Read the model definition and answer for the solid it produces. Units are mm, in the model's axes. Face numbers are marked on the shaded views. A direction names the side the tool comes from. Round coordinates to 2 decimals unless told otherwise and drop trailing zeros. Write each loop counter-clockwise with the first axis right and the second up, starting at its lowest first coordinate (ties: lowest second). Pieces come first, ordered by that corner, then holes. Notation, with made-up numbers: (3.5, 23.5) -> (12.5, 23.5) arc R33 ccw to (12.5, 60.5) -> close; hole circle Ø10 at (24.25, 84). An arc over 180 degrees is marked (long way). Return JSON: item names as keys, results as strings. Group by question number.
(1) For the marked faces 1 and 2, determine the directions among +Z, -Z, +X, -X, +Y, -Y from which every point of the face is accessible in a straight line to the end or side of a thin tool.
(2) Straight lines are drawn through the part: line 1 (Y direction, x = 0, z = 0.55); line 2 (X direction, y = 26, z = 0); line 3 (Y direction, x = -34.5, z = -0.65). For each, find the intervals that lie inside material, in ascending order.
(3) A cutting plane is placed at A-A on z = -0.75. Give the vertices of the cut face in (x, y), then the cut area to 3 significant figures.
(4) A cutting plane is placed at C-C on y = 22. State how many separate pieces and enclosed holes the cut face has, then the cut area to 3 significant figures.
(5) The mould has two halves that part along X. Classify the marked faces 3 and 4: released by +X, released by -X, zero draft, split by the parting line, or undercut.
(6) Given pin 1 (1 mm diameter, centred on y = -26, z = -2, fed in from -X); pin 2 (1 mm diameter, centred on y = -8, z = 0, fed in from -X); pin 3 (1.5 mm diameter, centred on y = -19.5, z = -2, fed in from +X), each flat-ended and moving along its own axis, determine where each tip first touches the part or whether it passes through.
(7) A cutting plane is placed at B-B on x = 0. Give the vertices of the cut face in (y, z), then the cut area to 3 significant figures.
```python
from build123d import *

# Parameters (mm, degrees)
CENTER_REACH             = 60.766
SKETCH3_R                = 7.5
CENTER_DIRECTION_2_REACH = 60.766
SPOKES_DEPTH             = 6
SKETCH5_R                = 2.75
HOLE_DEPTH               = 6


with BuildPart() as part:
    # Sketch2 → rim (revolve)
    with BuildSketch(Plane(origin=(0, 0, 0), x_dir=(1, 0, 0), z_dir=(0, 1, 0)), mode=Mode.PRIVATE) as rim_sk:
        with BuildLine():
            Line((41.5, -1.78), (41.5, -3))
            Line((41.5, -3), (38, -3))
            Line((38, -3), (38, 3))
            Line((38, 3), (41.5, 3))
            Line((41.5, 3), (41.5, 1.78))
            ThreePointArc((41.5, 1.78), (39.72, 0), (41.5, -1.78))
        make_face()
    revolve(rim_sk.sketch.rotate(Axis((0, 0, -19.925351406), (0, 0, 1)), 180), axis=Axis((0, 0, -19.925351406), (0, 0, 1)))


with BuildPart() as body_2:

    # center: up to this face of the body (flat: up to its plane)
    center_end = Plane(part.part.faces().sort_by_distance((40.326202743, 0, 3))[0])
    # Sketch3 → center (new, up to the picked face)
    with BuildSketch(Plane.XY, mode=Mode.PRIVATE) as center_sk1:
        with Locations(Location((0, 0, 0), (0, 0, 180))):
            Circle(SKETCH3_R)
    center_tool1 = split(extrude(center_sk1.sketch, amount=CENTER_REACH, mode=Mode.PRIVATE), bisect_by=center_end, keep=Keep.BOTH, mode=Mode.PRIVATE)
    add(center_tool1.solids().sort_by(Axis((0, 0, 0), (0, 0, 1)))[0])


    # center direction 2: up to this face of the body (flat: up to its plane)
    center_direction_2_end = Plane(part.part.faces().sort_by_distance((39.173797257, 0, -3))[0])
    # Sketch3 → center direction 2 (add, up to the picked face)
    with BuildSketch(Plane.XY, mode=Mode.PRIVATE) as center_direction_2_sk1:
        with Locations(Location((0, 0, 0), (0, 0, 180))):
            Circle(SKETCH3_R)
    center_direction_2_tool1 = split(extrude(center_direction_2_sk1.sketch, amount=-CENTER_DIRECTION_2_REACH, mode=Mode.PRIVATE), bisect_by=center_direction_2_end, keep=Keep.BOTH, mode=Mode.PRIVATE)
    add(center_direction_2_tool1.solids().sort_by(Axis((0, 0, 0), (0, 0, -1)))[0])


with BuildPart() as part_1:
    add(part.part)

    add(body_2.part)  # spokes merges body 2
    # Sketch4 → spokes (add)
    with BuildSketch(Plane.XY.offset(3)):
        Polygon((-1.454089233, 7.35769152), (23.049269408, 30.928550972), (25.47568141, 28.406146406), (3.06273149, 6.846143134), align=None)
        Polygon((5.644903153, 4.938123975), (38.309545548, -4.496977359), (37.338285116, -7.859514077), (7.460299618, 0.770668291), align=None)
        Polygon((7.098992386, -2.419567545), (15.26027614, -35.425528332), (11.862603706, -36.265660483), (4.397568127, -6.075474843), align=None)
        Polygon((1.454089233, -7.35769152), (-23.049269408, -30.928550972), (-25.47568141, -28.406146406), (-3.06273149, -6.846143134), align=None)
        Polygon((-5.644903153, -4.938123975), (-38.309545548, 4.496977359), (-37.338285116, 7.859514077), (-7.460299618, -0.770668291), align=None)
        Polygon((-7.098992386, 2.419567545), (-15.26027614, 35.425528332), (-11.862603706, 36.265660483), (-4.397568127, 6.075474843), align=None)
    extrude(amount=-SPOKES_DEPTH)

    # Sketch5 → hole (cut)
    with BuildSketch(Plane.XY.offset(3)):
        Circle(SKETCH5_R)
    extrude(amount=-HOLE_DEPTH, mode=Mode.SUBTRACT)


solid = part_1.part
```
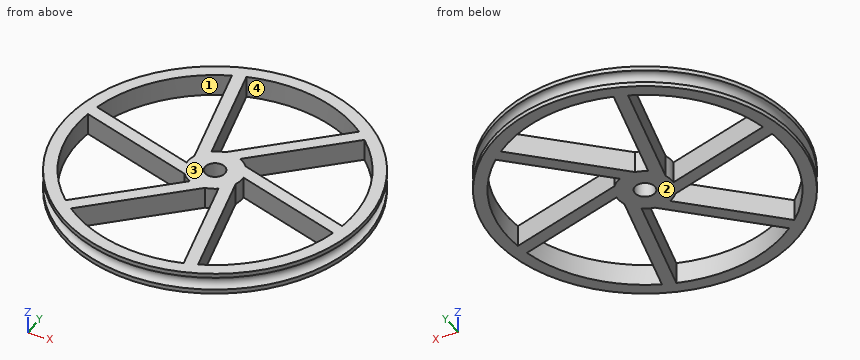
Checks:
{
 "1": {"face 1": "+Z, -Z", "face 2": "-Z, +X, -X, +Y, -Y"},
 "2": {"line 1": "y = -39.81 to -38, -8.76 to -2.75, 2.75 to 8.76, 38 to 39.81", "line 2": "x = -30.03 to -27.71, -12.93 to -9.32, 17.93 to 22.97, 27.71 to 30.03", "line 3": "y = -19.93 to -15.93, 3.4 to 7.04, 15.93 to 19.93"},
 "3": {"outline": "circle Ø79.77 at (0, 0); hole (-37.75, 4.34) arc R38 ccw to (-25.36, -28.3) -> (-3.06, -6.85) arc R7.5 cw to (-5.64, -4.94) -> close; hole (-37.19, 7.82) -> (-7.46, -0.77) arc R7.5 cw to (-7.1, 2.42) -> (-15.12, 34.86) arc R38 ccw to start; hole (-22.63, -30.53) arc R38 ccw to (11.82, -36.11) -> (4.4, -6.08) arc R7.5 cw to (1.45, -7.36) -> close; hole (-11.82, 36.11) -> (-4.4, 6.08) arc R7.5 cw to (-1.45, 7.36) -> (22.63, 30.53) arc R38 ccw to start; hole circle Ø5.5 at (0, 0); hole (3.06, 6.85) arc R7.5 cw to (5.64, 4.94) -> (37.75, -4.34) arc R38 ccw to (25.36, 28.3) -> close; hole (7.1, -2.42) -> (15.12, -34.86) arc R38 ccw to (37.19, -7.82) -> (7.46, 0.77) arc R7.5 cw to start", "area": "1,280 mm^2"},
 "4": {"separate pieces": "4", "enclosed holes": "0", "area": "90.6 mm^2"},
 "5": {"face 3": "zero draft", "face 4": "undercut"},
 "6": {"pin 1": "stops at x = -32.74", "pin 2": "stops at x = -39.01", "pin 3": "stops at x = 37.02"},
 "7": {"outline": "(-41.5, -3) -> (-38, -3) -> (-38, 3) -> (-41.5, 3) -> (-41.5, 1.78) arc R1.78 cw to (-41.5, -1.78) -> close; (-8.76, -3) -> (-2.75, -3) -> (-2.75, 3) -> (-8.76, 3) -> close; (2.75, -3) -> (8.76, -3) -> (8.76, 3) -> (2.75, 3) -> close; (38, -3) -> (41.5, -3) -> (41.5, -1.78) arc R1.78 cw to (41.5, 1.78) -> (41.5, 3) -> (38, 3) -> close", "area": "104 mm^2"}
}
